Autodesk Inventor part; units mm, degrees
ref_plane "YZ Plane" through (0, 0, 0) normal (1, 0, 0) x (0, 1, 0)
ref_plane "XZ Plane" through (0, 0, 0) normal (0, 1, 0) x (-1, 0, 0)
ref_plane "XY Plane" through (0, 0, 0) normal (0, 0, 1) x (1, 0, 0)
sketch "スケッチ1" plane through (0, 0, 0) normal (1, 0, 0) x (0, 1, 0)
  line L0 (0, 0) -> (30, 0)
  line L1 (30, 0) -> (30, -43)
  line L2 (30, -43) -> (0, -43)
  line L3 (0, -43) -> (0, 0)
  circle A0 centre (15, -5) radius 1.6
  circle A1 centre (15, -38) radius 1.6
  line L4 (28.75, -18.3) -> (26.18, -18.3)
  line L5 (26.18, -18.3) -> (26.18, -24.7)
  line L6 (26.18, -24.7) -> (28.75, -24.7)
  line L7 (28.75, -24.7) -> (28.75, -18.3)
  line L8 (30, -21.5) -> (0, -21.5)
  line L9 (23.67, -18.3) -> (21.1, -18.3)
  line L10 (21.1, -24.7) -> (23.67, -24.7)
  line L11 (23.67, -24.7) -> (23.67, -18.3)
  line L12 (21.1, -18.3) -> (21.1, -24.7)
  line L13 (18.59, -18.3) -> (16.02, -18.3)
  line L14 (16.02, -24.7) -> (18.59, -24.7)
  line L15 (18.59, -24.7) -> (18.59, -18.3)
  line L16 (16.02, -18.3) -> (16.02, -24.7)
  line L17 (13.51, -18.3) -> (10.94, -18.3)
  line L18 (10.94, -24.7) -> (13.51, -24.7)
  line L19 (13.51, -24.7) -> (13.51, -18.3)
  line L20 (10.94, -18.3) -> (10.94, -24.7)
  line L21 (8.43, -18.3) -> (5.86, -18.3)
  line L22 (5.86, -24.7) -> (8.43, -24.7)
  line L23 (8.43, -24.7) -> (8.43, -18.3)
  line L24 (5.86, -18.3) -> (5.86, -24.7)
  line L25 (3.35, -18.3) -> (0.78, -18.3)
  line L26 (0.78, -24.7) -> (3.35, -24.7)
  line L27 (3.35, -24.7) -> (3.35, -18.3)
  line L28 (0.78, -18.3) -> (0.78, -24.7)
  line L29 (30, -24.7) -> (0, -24.7)
  line L30 (0, -24.7) -> (0, -18.3)
  line L31 (0, -18.3) -> (30, -18.3)
  line L32 (30, -18.3) -> (30, -24.7)
  point P0 (0, -24.7)
  dimension "d0" = 30
  dimension "d1" = 43
  dimension "d2" = 3.2
  dimension "d3" = 3.2
  dimension "d4" = 5
  dimension "d5" = 15
  dimension "d6" = 15
  dimension "d7" = 5
  dimension "d8" = 2.57
  dimension "d9" = 6.4
  dimension "d10" = 3.2
  dimension "d11" = 1.25
  dimension "d14" = 5.08
  dimension "d22" = 0
  dimension "d23" = 0
extrude "押し出し1" add sketch "スケッチ1" along normal blind 5 contours L0 L1 L31 L4 L9 L13 L17 L21 L25 L3 | L31 L28 L8 L3 | L1 L8 L7 L31 | L8 L28 L29 L3 | L1 L29 L7 L8 | L29 L26 L22 L18 L14 L10 L6 L1 L2 L3 | L31 L24 L8 L27 | L5 L8 L11 L31 | L8 L24 L29 L27 | L5 L29 L11 L8 | L31 L20 L8 L23 | L12 L8 L15 L31 | L8 L20 L29 L23 | L12 L29 L15 L8 | L31 L16 L8 L19 | L8 L16 L29 L19
fillet "フィレット1" radius 2 4 edges at (2.5, 30, 0) (2.5, 0, 0) (2.5, 0, -43) (2.5, 30, -43)
extrude "押し出し2" cut sketch "スケッチ1" along normal blind 1 contours L31 L28 L8 L3 | L1 L8 L7 L31 | L8 L28 L29 L3 | L25 L27 L8 L28 | L1 L29 L7 L8 | L7 L8 L5 L4 | L8 L27 L26 L28 | L31 L24 L8 L27 | L7 L6 L5 L8 | L5 L8 L11 L31 | L8 L24 L29 L27 | L21 L23 L8 L24 | L5 L29 L11 L8 | L11 L8 L12 L9 | L8 L23 L22 L24 | L31 L20 L8 L23 | L11 L10 L12 L8 | L12 L8 L15 L31 | L8 L20 L29 L23 | L17 L19 L8 L20 | L12 L29 L15 L8 | L15 L8 L16 L13 | L8 L19 L18 L20 | L31 L16 L8 L19 | L15 L14 L16 L8 | L8 L16 L29 L19
equation "\"d6\" = d5"
equation "\"d7\" = d4"
properties part number "dribl-v3-3DP-3" material "ABS プラスチック"
Read the model definition and answer for the solid it produces. Units are mm, in the model's axes. A direction names the side the tool comes from. Give positions to 0.01 mm unless a question says otherwise; leave off trailing zeros. Order: outer loops, then holes, each group sorted by start corner. A loop starts at its lowest first (then second) coordinate and runs counter-clockwise, first axis right, second up. Notation, with made-up numbers: (36.5, 72.5) -> (82.5, 72.5) arc R21 cw to (82.5, 103.5) -> close; hole circle Ø6 at (0.5, 44). An arc over 180 degrees is marked (long way). One line per item, written item: value. Start each with the question number.
(1) A tool of negligible diameter and unlimited length cuts with its end or side. For faces 1 (the flat face through (2, 30, -21)), 2 (the flat face through (3, 28.75, -22)), 3 (the flat face through (1, 25, -21)), from which of +Z, -Z, +X, -X, +Y, -Y can it reach the whole face along a straight path? Write none if from no direction.
(2) The part is cut by section D-D (z = -38). Determine the outline of the cut face in (x, y), and give its area (3 significant figures).
(3) The part is cut by section B-B (y = 27). Determine the outline of the cut face in (x, z).
(4) Straight lines are drawn through the part: L1, parallel to Z at x = 3.35, y = 15; L2, parallel to Z at x = 2.3, y = 7; L3, parallel to Z at x = 2.9, y = 14.5. For each, find the intervals that lie inside material, in ascending order.
(5) A flat-ended cylindrical pin translates along its axis: P1, Ø2, axis at y = 20, z = -20.5, coming from the -X side. Find the tip coordinate at first contact, or state that the pin passes through.
(6) The part is cut by section A-A (y = 15). Determine the outline of the cut face in (x, z), and give its area (3 significant figures).
(7) For a pull along Y with two mould halves and no side action, classify faces 4 (the flat face through (5, 15, -21)), 5 (the cylindrical face through (2.54, 29.4, -42.43)), 6 (the flat face through (3, 26.18, -21)) as released by +Y, released by -Y, zero draft, split by the parting line, or undercut.
(8) The part is cut by section C-C (x = 2.75). State how many separate pieces and enclosed holes the cut face has, and give its area (3 significant figures).
Taken from the geometry:
1. face 1: +Z, -Z, +X, -X, +Y
1. face 2: +X, -X
1. face 3: -X, +Y, -Y
2. outline: (0, 0) -> (5, 0) -> (5, 13.4) -> (0, 13.4) -> close; (0, 16.6) -> (5, 16.6) -> (5, 30) -> (0, 30) -> close
2. area: 134 mm^2
3. outline: (0, -43) -> (5, -43) -> (5, -24.7) -> (0, -24.7) -> close; (0, -18.3) -> (5, -18.3) -> (5, 0) -> (0, 0) -> close
4. L1: -43 to -39.6, -36.4 to -6.6, -3.4 to 0
4. L2: -43 to -24.7, -18.3 to 0
4. L3: -43 to -39.52, -36.48 to -6.52, -3.48 to 0
5. P1: x = 1
6. outline: (0, -43) -> (5, -43) -> (5, -39.6) -> (0, -39.6) -> close; (0, -36.4) -> (5, -36.4) -> (5, -6.6) -> (0, -6.6) -> (0, -18.3) -> (1, -18.3) -> (1, -24.7) -> (0, -24.7) -> close; (0, -3.4) -> (5, -3.4) -> (5, 0) -> (0, 0) -> close
6. area: 177 mm^2
7. face 4: zero draft
7. face 5: released by +Y
7. face 6: undercut
8. separate pieces: 1
8. enclosed holes: 8
8. area: 1,170 mm^2
